The listing builds one solid part. Answer for the finished solid, in the listing's coordinates (mm). Face numbers are marked on the shaded views. A direction names the side the tool comes from. Round coordinates to 2 decimals unless told otherwise and drop trailing zeros. Loops run counter-clockwise (first coordinate to the right, second up) from the corner with the lowest first, then second, coordinate; pieces in that order, holes last. Notation, with made-up numbers: M 88,-1.5 L 134,-1.5 A19 ccw 134,19.5 Z; hole C 14.5,29 d6. An arc over 180 degrees is marked long. Answer as a JSON object with one key per item and string values.
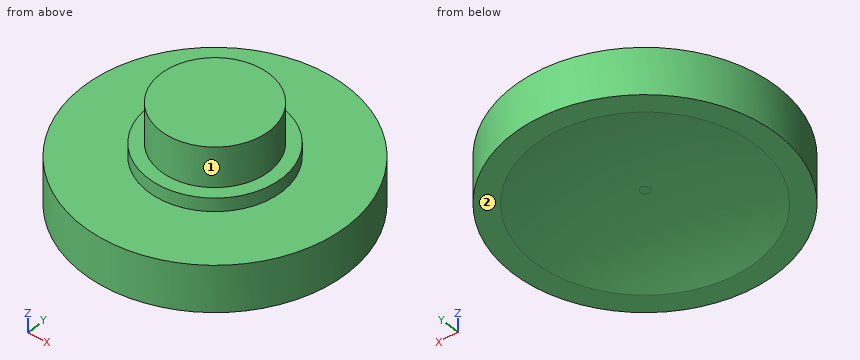
```python
from build123d import *

# Parameters (mm, degrees)
F0_R     = 9.8592181747
F1_DEPTH = 3.5
F2_R     = 5
F3_DEPTH = 1
F4_R     = 4.05
F5_DEPTH = 3
F6_R     = 8.2811029309
F7_DEPTH = 1


# Not quite as in the source:
# - a fillet or chamfer that OpenCascade refuses, or shapes differently, is made with other operations: its cross-section is extruded or revolved along the edge and cut away or added


with BuildPart() as f1:
    # F0 (on Top) → F1 (new body)
    with BuildSketch(Plane.XY):
        Circle(F0_R)
    extrude(amount=F1_DEPTH)

    # F2 (on face) → F3 (join)
    with BuildSketch(Plane.XY.offset(3.5)):
        Circle(F2_R)
    extrude(amount=F3_DEPTH)

    # F4 (on face) → F5 (join)
    with BuildSketch(Plane.XY.offset(4.5)):
        Circle(F4_R)
    extrude(amount=F5_DEPTH)

    # F6 (on face) → F7 (cut)
    with BuildSketch(Plane(origin=(0, 0, 0), x_dir=(1, 0, 0), z_dir=(0, 0, -1))):
        Circle(F6_R)
    extrude(amount=-F7_DEPTH, mode=Mode.SUBTRACT)

    # F8: fillet of radius 32 on 1 edges, made by hand

    # F8_s1 → F8_t2 (revolve)
    with BuildSketch(Plane.XZ):
        with BuildLine():
            ThreePointArc((8.2811029309, 0), (4.3438489977, 0.7490157328), (0.3438489977, 1))
            Line((0.3438489977, 1), (8.2811029309, 1))
            Line((8.2811029309, 1), (8.2811029309, 0))
        make_face()
    revolve(axis=Axis((0, 0, 1), (0, 0, -1)))


solid = f1.part
```
Item 1: The part is cut by section A-A (z = 3.25). Give the vertices of the cut face in (x, y).
Values follow:
{"outline": "C 0,0 d19.72"}
Item 2: Flat-ended cylindrical pins translate along their axes: P1, Ø3, axis at x = 6, z = 4, coming from the -Y side; P2, Ø2, axis at x = -4.5, y = 5.5, coming from the +Z side; P3, Ø2, axis at y = 7, z = 3, coming from the -X side. Find the tip coordinate at first contact, or state that the pin passes through.
Values follow:
{"P1": "y = -8.73", "P2": "z = 3.5", "P3": "x = -7.82"}
Item 3: Which of the six approach directions +Z, -Z, +X, -X, +Y, -Y give full straight-line access (tool end or side, diameter ignored) to the marked faces 1 and 2?
Values follow:
{"face 1": "+Z", "face 2": "-Z, +X, -X, +Y, -Y"}
Item 4: The part is cut by section B-B (z = 5). Give the vertices of the cut face in (x, y), then the cut area to 3 significant figures.
Values follow:
{"outline": "C 0,0 d8.1", "area": "51.5 mm^2"}
Item 5: Straight lines are drawn through the part: line 1 (Z direction, x = -3, y = -8); line 2 (Y direction, x = 8.5, z = 1.5); line 3 (X direction, y = 8, z = 1.75). For each, find the intervals that lie inside material, in ascending order.
Values follow:
{"line 1": "0 to 3.5", "line 2": "-5 to 5", "line 3": "-5.76 to 5.76"}
